The listing builds one solid part. Answer for the finished solid, in the listing's coordinates (mm). A direction names the side the tool comes from. Give positions to 0.01 mm unless a question says otherwise; leave off trailing zeros. Write each loop counter-clockwise with the first axis right and the second up, starting at its lowest first coordinate (ties: lowest second). Pieces come first, ordered by that corner, then holes. Notation, with made-up numbers: (3.5, 40.5) - (27.5, 40.5) arc R19 ccw to (27.5, 57.5) - close; hole circle Ø3 at (10, -40). An arc over 180 degrees is marked (long way). Return JSON: item names as keys, results as strings.
from build123d import *

# Parameters (mm, degrees)
EXTRUDE_1_DEPTH     = 20
SKETCH_13_R         = 2
CUT_EXTRUDE_7_DEPTH = 51
SKETCH_16_R         = 2
CUT_EXTRUDE_8_DEPTH = 51
FILLET_2_R          = 10


with BuildPart() as part:
    # 草图2 → 凸台-拉伸1 (new body)
    with BuildSketch(Plane.XY):
        Polygon((0, 0), (0, -4), (-18.7435877, -4), (-84.7435877, -50), (-106, -50), (-106, -46), (-86, -46), (-20, 0), align=None)
    extrude(amount=EXTRUDE_1_DEPTH)

    # 草图13 → 切除-拉伸7 (cut, through all)
    with BuildSketch(Plane(origin=(0, 0, 0), x_dir=(1, 0, 0), z_dir=(0, 1, 0))):
        with Locations((-10, -10)):
            Circle(SKETCH_13_R)
    extrude(amount=-CUT_EXTRUDE_7_DEPTH, mode=Mode.SUBTRACT)

    # 草图16 → 切除-拉伸8 (cut, through all)
    with BuildSketch(Plane.XZ.offset(50)):
        with Locations((-96, 10)):
            Circle(SKETCH_16_R)
    extrude(amount=-CUT_EXTRUDE_8_DEPTH, mode=Mode.SUBTRACT)

    # 圆角2
    fillet_2_edges = [part.edges().sort_by_distance(p)[0] for p in [
        (-18.7435877, -4, 10),
        (-86, -46, 10),
    ]]
    fillet(fillet_2_edges, radius=FILLET_2_R)


solid = part.part
Item 1: Consider L1, parallel to Z at x = -96, y = -47; L2, parallel to Y at x = -90.5, z = 15; L3, parallel to X at y = -2.1, z = 10. Determine where each line is inside the solid, lowest interval first.
Answer below:
{"L1": "z = 0 to 8, 12 to 20", "L2": "y = -50 to -46", "L3": "x = -23.01 to -12, -8 to 0"}
Item 2: A cutting plane is placed at D-D on x = -36.5. Determine the outline of the cut face in (y, z), then the cut area to 3 significant figures.
Answer below:
{"outline": "(-16.38, 0) - (-11.5, 0) - (-11.5, 20) - (-16.38, 20) - close", "area": "97.5 mm²"}
Item 3: For faces 1 (the face through (-106, -48, 10)), 2 (the face through (-100, -46, 10)), 3 (the face through (-7.7, -4, 9.9)), determine the directions among +Z, -Z, +X, -X, +Y, -Y from which every point of the face is accessible in a straight line to the end or side of a thin tool.
Answer below:
{"face 1": "+Z, -Z, -X, +Y, -Y", "face 2": "+Z, -Z, -X, +Y", "face 3": "+Z, -Z, +X, -Y"}
Item 4: A cutting plane is placed at B-B on x = -10. Determine the outline of the cut face in (y, z).
Answer below:
{"outline": "(-4, 0) - (0, 0) - (0, 8) - (-4, 8) - close; (-4, 12) - (0, 12) - (0, 20) - (-4, 20) - close"}
Item 5: The mould has two halves that part along Z. Classify faces 4 (the face through (-53, -25, 0)), 5 (the face through (-94.092, -48.028, 10.601)), 6 (the face through (-10, -2, 8)), 7 (the face through (0, -2, 10)): +Z half, -Z half, draft (parallel to the pull), parting line (faces both ways), or undercut.
Answer below:
{"face 4": "-Z half", "face 5": "undercut", "face 6": "undercut", "face 7": "draft"}
Item 6: Flat-ended cylindrical pins translate along their axes: P1, Ø5, axis at x = -75, z = 5, coming from the -Y side; P2, Ø5, axis at x = -68.5, y = -42.5, coming from the +Z side; P3, Ø4, axis at x = -71, z = 13, coming from the +Y side; P4, Ø4.5, axis at x = -96, z = 10, coming from the +Y side. Find the tip coordinate at first contact, or state that the pin passes through.
Answer below:
{"P1": "stops at y = -44.95", "P2": "passes through", "P3": "stops at y = -34.15", "P4": "stops at y = -46"}
Item 7: A cutting plane is placed at C-C on z = 5.75. Determine the outline of the cut face in (x, y).
Answer below:
{"outline": "(-106, -50) - (-84.74, -50) - (-21.32, -5.8) arc R10 cw to (-15.6, -4) - (0, -4) - (0, 0) - (-20, 0) - (-83.42, -44.2) arc R10 cw to (-89.14, -46) - (-106, -46) - close"}
Item 8: A cutting plane is placed at A-A on z = 10. Determine the outline of the cut face in (x, y).
Answer below:
{"outline": "(-106, -50) - (-98, -50) - (-98, -46) - (-106, -46) - close; (-94, -50) - (-84.74, -50) - (-21.32, -5.8) arc R10 cw to (-15.6, -4) - (-12, -4) - (-12, 0) - (-20, 0) - (-83.42, -44.2) arc R10 cw to (-89.14, -46) - (-94, -46) - close; (-8, -4) - (0, -4) - (0, 0) - (-8, 0) - close"}
